```python
from build123d import *

# Parameters (mm, degrees)
SKETCH1_R           = 4.5
BOSS_EXTRUDE1_DEPTH = 3
BOSS_EXTRUDE2_DEPTH = 2
SKETCH3_R           = 1
CUT_EXTRUDE1_DEPTH  = 2
SKETCH4_R           = 1.5
CUT_EXTRUDE3_DEPTH  = 32
CHAMFER1_SIZE       = 2
CUT_EXTRUDE4_DEPTH  = 32
FILLET1_R           = 3
SKETCH6_R           = 1.5
CUT_EXTRUDE5_DEPTH  = 2


with BuildPart() as part:
    # Sketch1 → Boss-Extrude1 (new body)
    with BuildSketch(Plane(origin=(0, 0, 0), x_dir=(1, 0, 0), z_dir=(0, 1, 0))):
        with Locations(Location((0, 0, 0), (0, 0, 270))):
            Circle(SKETCH1_R)
    extrude(amount=BOSS_EXTRUDE1_DEPTH)

    # Sketch2 → Boss-Extrude2 (add)
    with BuildSketch(Plane(origin=(0, 3, 0), x_dir=(1, 0, 0), z_dir=(0, 1, 0))):
        with BuildLine():
            Line((4.479718811, 0), (4.479718811, -14))
            ThreePointArc((4.479718811, -14), (0, -18.479718811), (-4.479718811, -14))
            Line((-4.479718811, -14), (-4.479718811, 0))
            ThreePointArc((-4.479718811, 0), (0, 4.479718811), (4.479718811, 0))
        make_face()
    extrude(amount=BOSS_EXTRUDE2_DEPTH)

    # Sketch3 → Cut-Extrude1 (cut)
    with BuildSketch(Plane(origin=(0, 5, 0), x_dir=(1, 0, 0), z_dir=(0, 1, 0))):
        with Locations(Location((0, -14, 0), (0, 0, 270))):
            Circle(SKETCH3_R)
    extrude(amount=-CUT_EXTRUDE1_DEPTH, mode=Mode.SUBTRACT)

    # Sketch4 → Cut-Extrude3 (cut)
    with BuildSketch(Plane(origin=(0, 5, 0), x_dir=(1, 0, 0), z_dir=(0, 1, 0))):
        with Locations(Location((0, 0, 0), (0, 0, 270))):
            Circle(SKETCH4_R)
    extrude(amount=-CUT_EXTRUDE3_DEPTH, mode=Mode.SUBTRACT)

    # Chamfer1
    chamfer1_edges = [part.edges().sort_by_distance(p)[0] for p in [
        (0, 5, -1.5),
    ]]
    chamfer(chamfer1_edges, length=CHAMFER1_SIZE)

    # Sketch5 → Cut-Extrude4 (cut)
    with BuildSketch(Plane(origin=(0, 5, 0), x_dir=(1, 0, 0), z_dir=(0, 1, 0))):
        Polygon((4.479718811, 0), (2.781543996, -17.511537216), (5.759954013, -17.140136672), (7.823781183, -10.648462117), align=None)
        Polygon((-4.479718811, 0), (-2.781543996, -17.511537216), (-11.97019759, -15.320216349), align=None)
    extrude(amount=-CUT_EXTRUDE4_DEPTH, mode=Mode.SUBTRACT)

    # Fillet1
    # the kernel refuses this fillet: 3 mm, written as the material it takes off along each edge
    with BuildSketch(Plane(origin=(-2.781543996, 12.615972723, 17.511537216), x_dir=(0.9482948551929795, 0, 0.31739071759351406), z_dir=(0, -1, 0))) as fillet1_piece_1:
        with BuildLine():
            CenterArc((2.026328718, -2.82125448), FILLET1_R, 70.121899875, 85.833982954)
            Line((-0.713367294, -1.59893465), (0, 0))
            ThreePointArc((0, 0), (1.523194545, 0.26690989), (3.046389089, 0))
        make_face()
    extrude(amount=17.231945445, mode=Mode.SUBTRACT)
    with BuildSketch(Plane(origin=(2.781543996, 12.615972723, 17.511537216), x_dir=(-0.9482948551929786, 0, 0.3173907175935166), z_dir=(0, -1, 0))) as fillet1_piece_2:
        with BuildLine():
            CenterArc((2.026328718, 2.82125448), FILLET1_R, 204.044117171, 85.833982954)
            Line((-0.713367294, 1.59893465), (0, 0))
            ThreePointArc((0, 0), (1.523194545, -0.26690989), (3.046389089, 0))
        make_face()
    extrude(amount=17.231945445, mode=Mode.SUBTRACT)

    # Sketch6 → Cut-Extrude5 (cut)
    with BuildSketch(Plane(origin=(0, 5, 0), x_dir=(1, 0, 0), z_dir=(0, 1, 0))):
        with Locations(Location((0, -14, 0), (0, 0, 270))):
            Circle(SKETCH6_R)
    extrude(amount=-CUT_EXTRUDE5_DEPTH, mode=Mode.SUBTRACT)


solid = part.part
```
CAD build for the part. Positions are in the model's coordinates, mm. A direction names the side the tool comes from. Coordinates: 2 decimals unless noted, no trailing zeros. Order: outer loops, then holes, each group sorted by start corner. A loop starts at its lowest first (then second) coordinate and runs counter-clockwise, first axis right, second up. Notation, with made-up numbers: (88, -14.5) - (95, -14.5) arc R21 ccw to (95, 20.5) - close; hole circle Ø8 at (-22, 11.5). An arc over 180 degrees is marked (long way). Answer in a Markdown table with one row per item.
1. Slice it at C-C, the plane z = 14. List the corners of the cut face in (x, y).
Answer:
| item | result |
|---|---|
| outline | (-3.12, 3) - (-1.5, 3) - (-1.5, 5) - (-3.12, 5) - close; (1.5, 3) - (3.12, 3) - (3.12, 5) - (1.5, 5) - close |
2. Slice it at B-B, the plane y = 2.2. List the corners of the cut face in (x, z), then the cut area to 3 significant figures.
Answer:
| item | result |
|---|---|
| outline | (-4.5, 0.04) arc R4.5 ccw (long way) to (4.5, 0.06) - (4.48, 0) - (4.38, 1.04) arc R4.5 ccw to (-4.38, 1.04) - (-4.48, 0) - close; hole circle Ø3 at (0, 0) |
| area | 56.5 mm² |
3. Drill centre lines: L1, parallel to Y at x = 0.75, z = 8.75; L2, parallel to X at y = 3.75, z = -1.5; L3, parallel to Z at x = 2.25, y = 4.75. Where is each one in solid material? Low to high. Write a range as from..to.
Answer:
| item | result |
|---|---|
| L1 | 3..5 |
| L2 | -4.22..-1.68, 1.68..4.22 |
| L3 | -3.87..-2.35, 2.35..17.42 |
4. Pull direction X, two halves, no side cores. Call faces 1 (the face through (0.45, 1.52, 1.43)), 2 (the face through (-0.1, 1.5, 4.5)), 3 (the face through (0.07, 4.01, 12.5)), 4 (the face through (0, 5, 7)): +X half, -X half, draft (parallel to the pull), parting line (faces both ways), or undercut.
Answer:
| item | result |
|---|---|
| face 1 | undercut |
| face 2 | parting line |
| face 3 | undercut |
| face 4 | draft |
5. 3-axis set-ups, long thin cutter, end or side, ignore diameter. For faces 5 (the face through (-1.97, 4.01, 17.71)), 6 (the face through (-0.1, 3.99, -4.48)): which of +Z, -Z, +X, -X, +Y, -Y reach the whole face in a straight line?
Answer:
| item | result |
|---|---|
| face 5 | +Z, -X, +Y, -Y |
| face 6 | -Z, +Y |
6. Flat gauge pins, fed straight in: P1, Ø3, axis at y = 4, z = 11.5, coming from the +X side; P2, Ø2, axis at x = -0.5, y = 1, coming from the +Z side; P3, Ø2, axis at y = 4, z = -2, coming from the +X side; P4, Ø2.5, axis at x = 0, z = 0, coming from the +Y side. Where does each tip first touch, or does it go through?
Answer:
| item | result |
|---|---|
| P1 | x = 3.51 |
| P2 | z = 4.5 |
| P3 | x = 4.37 |
| P4 | through |
7. Slice it at A-A, the plane y = 4.1. List the corners of the cut face in (x, z), then the cut area to 3 significant figures.
Answer:
| item | result |
|---|---|
| outline | (-4.48, 0) arc R4.48 ccw to (4.48, 0) - (2.95, 15.77) arc R3 ccw to (0, 18.48) arc R3 ccw to (-2.95, 15.77) - close; hole circle Ø5.2 at (0, 0); hole circle Ø3 at (0, 14) |
| area | 133 mm² |
